Geometry: final body of the model. Coordinates: model frame, mm. A direction names the side the tool comes from. Coordinates: 2 decimals unless noted, no trailing zeros. Write each loop counter-clockwise with the first axis right and the second up, starting at its lowest first coordinate (ties: lowest second). Pieces come first, ordered by that corner, then holes.
from build123d import *

# Parameters (mm, degrees)
F3_START = -4.5
F3_DEPTH = 4


with BuildPart() as f1:
    # F0 (on Right) → F1 (revolve)
    with BuildSketch(Plane.YZ):
        Polygon((26, 0), (2, 0), (2, -2), (0, -2), (0, -14), (10, -14), (10, -12.5), (18.5, -12.5), (18.5, -6), (21, -8.5), (23.5, -6), (26, -8.5), (28.5, -6), (31, -8.5), (33.5, -6), (36, -8.5), (36, -4.5), (33.5, -2), (31, -4.5), (28.5, -2), (26, -4.5), align=None)
        with BuildLine():
            Line((10, -14), (0, -14))
            Line((0, -14), (0, -17))
            ThreePointArc((0, -17), (5.2201532545, -16.2338441815), (10, -14))
        make_face()
    revolve(axis=Axis((0, 0, -6.3047250733), (0, 0, -1)))

    # F2 (on face) → F3 (join)
    with BuildSketch(Plane.XY.offset(F3_START)):
        with BuildLine():
            ThreePointArc((-33.2049675533, -13.5), (-36, 0), (-33.2049675533, 13.5))
            Line((-33.2049675533, 13.5), (-70.5000009461, 13.5))
            ThreePointArc((-70.5000009461, 13.5), (-84, 0), (-70.5000009461, -13.5))
            Line((-70.5000009461, -13.5), (-33.2049675533, -13.5))
        make_face()
        with BuildLine():
            ThreePointArc((-70.5, -9), (-79.5, 0), (-70.5, 9))
            Line((-70.5, 9), (-63.5, 9))
            ThreePointArc((-63.5, 9), (-57.1360389693, 6.3639610307), (-54.5, 0))
            ThreePointArc((-54.5, 0), (-57.1360389693, -6.3639610307), (-63.5, -9))
            Line((-63.5, -9), (-70.5, -9))
        make_face(mode=Mode.SUBTRACT)
        with BuildLine():
            Line((33.2049675533, -13.5), (70.5000009461, -13.5))
            ThreePointArc((70.5000009461, -13.5), (84, 0), (70.5000009461, 13.5))
            Line((70.5000009461, 13.5), (33.2049675533, 13.5))
            ThreePointArc((33.2049675533, 13.5), (36, 0), (33.2049675533, -13.5))
        make_face()
        with BuildLine():
            Line((63.5, 9), (70.5, 9))
            ThreePointArc((70.5, 9), (76.8639610307, 6.3639610307), (79.5, 0))
            ThreePointArc((79.5, 0), (76.8639610307, -6.3639610307), (70.5, -9))
            Line((70.5, -9), (63.5, -9))
            ThreePointArc((63.5, -9), (54.5, 0), (63.5, 9))
        make_face(mode=Mode.SUBTRACT)
    extrude(amount=-F3_DEPTH)


solid = f1.part
Item 1: Set-up query: faces 1 (the flat face through (52, 13.5, -6)), 2 (the flat face through (0, 0, -2)), 3 (the cylindrical face through (54.502, -0.198, -6.472)), 4 (the flat face through (-52, -13.5, -6)). Return all of +Z, -Z, +X, -X, +Y, -Y with unobstructed straight access to the full face (end or side cutting, diameter ignored); none if empty.
Derived:
face 1: +Z, -Z, +X, +Y
face 2: +Z
face 3: +Z, -Z
face 4: +Z, -Z, -X, -Y
Item 2: Section A-A, the plane x = 58. Output: boundary loops of the cut face in (y, z).
Derived:
outline: (-13.5, -8.5) - (-7.12, -8.5) - (-7.12, -4.5) - (-13.5, -4.5) - close; (7.12, -8.5) - (13.5, -8.5) - (13.5, -4.5) - (7.12, -4.5) - close
Item 3: Material intervals for probe 1 along X at (y, z) = (0, -1.35); probe 2 along Y at (x, z) = (-65.5, -4.75); probe 3 along X at (y, z) = (16, -3), sorted ascending.
Derived:
probe 1: x = -26 to -2, 2 to 26
probe 2: y = -13.5 to -9, 9 to 13.5
probe 3: x = -30.57 to -28.29, -24.78 to -22.37, -20.49 to 20.49, 22.37 to 24.78, 28.29 to 30.57
Item 4: Pin query (flat end, axial travel): pin 1 (10 mm diameter, centred on y = -3.5, z = -2.5, fed in from +X); pin 2 (1.2 mm diameter, centred on x = 66, z = -7, fed in from +Y); pin 3 (4.5 mm diameter, centred on x = -60, z = -7, fed in from -Y); pin 4 (10 mm diameter, centred on y = -25, z = -10, fed in from +X). Return the tip coordinate at first contact, or that it passes through.
Derived:
pin 1: stops at x = 84
pin 2: stops at y = 13.5
pin 3: stops at y = -13.5
pin 4: stops at x = 29.78
Item 5: Section D-D, the plane x = 41. Output: boundary loops of the cut face in (y, z), plus the area to 3 significant figures.
Derived:
outline: (-13.5, -8.5) - (13.5, -8.5) - (13.5, -4.5) - (-13.5, -4.5) - close
area: 108 mm2
Item 6: Section B-B, the plane z = -11. Output: boundary loops of the cut face in (x, y).
Derived:
outline: circle Ø37 at (0, 0)
Item 7: Section C-C, the plane x = -59. Output: boundary loops of the cut face in (y, z), plus the area to 3 significant figures.
Derived:
outline: (-13.5, -8.5) - (-7.79, -8.5) - (-7.79, -4.5) - (-13.5, -4.5) - close; (7.79, -8.5) - (13.5, -8.5) - (13.5, -4.5) - (7.79, -4.5) - close
area: 45.6 mm2
